Part model, mm, in its own coordinate system. A direction names the side the tool comes from. Round coordinates to 2 decimals unless told otherwise and drop trailing zeros. Write each loop counter-clockwise with the first axis right and the second up, starting at its lowest first coordinate (ties: lowest second). Pieces come first, ordered by that corner, then holes.
1) Drill centre lines: L1, parallel to Z at x = -0.5, y = -14.5; L2, parallel to Y at x = -0.7, z = 54.5; L3, parallel to Z at x = 1.3, y = -5.5. Where is each one in solid material? Low to high.
2) Saw through at B-B on z = 48. Write the cut outline in (x, y), and give its area (3 significant figures).
3) Flat gauge pins, fed straight in: pin 1 (1.6 mm diameter, centred on y = -5.02, z = 28.49, fed in from -X); pin 2 (1 mm diameter, centred on x = 1, y = 53, fed in from -Z); pin 3 (1 mm diameter, centred on x = -1, z = -19, fed in from +Y); pin 4 (1 mm diameter, centred on x = 2, z = -23.5, fed in from -Y). Where does each tip first touch, or does it go through?
4) Saw through at A-A on y = -34. Write the cut outline in (x, z).
5) Saw through at C-C on y = 45. Write the cut outline in (x, z), and give its area (3 significant figures).
6) Which spindle directions (+Z, -Z, +X, -X, +Y, -Y) get a long thin tool onto all of the face, cutting with end or side? Do faces 1 (the flat face through (0.042, -64.765, -1.144)), 2 (the cylindrical face through (0.042, 7.046, 60.318)), 3 (the flat face through (0.042, 23.317, -13.135)). Say none if no direction does.
```python
from build123d import *

# Parameters (mm, degrees)
SKETCH1_R                = 59
EXTRUDE1_DEPTH           = 3
EXTRUDE2_DEPTH           = 3
CIRPATTERN1_COUNT        = 6
F_2_0_2_DIAMETER_HOLE1_D = 2
F_2_0_2_DIAMETER_HOLE3_D = 2
F_2_0_2_DIAMETER_HOLE4_D = 2
CIRPATTERN2_COUNT        = 6
CIRPATTERN3_COUNT        = 5
CIRPATTERN3_ANGLE        = 240


with BuildPart() as part:
    # Sketch1 → Extrude1 (new, symmetric)
    with BuildSketch(Plane(origin=(0, 0, 0), x_dir=(0, 0, -1), z_dir=(1, 0, 0))):
        Circle(SKETCH1_R)
        Polygon((28.485808967, 5.022816688), (9.893017633, 27.180842557), (-18.592791334, 22.158025869), (-28.485808967, -5.022816688), (-9.893017633, -27.180842557), (18.592791334, -22.158025869), align=None, mode=Mode.SUBTRACT)
    extrude(amount=EXTRUDE1_DEPTH, both=True)

    # Sketch2 → Extrude2 (add, symmetric)
    with BuildSketch(Plane(origin=(0, 0, 0), x_dir=(0, 0, -1), z_dir=(1, 0, 0))):
        with BuildLine():
            Line((-2, 67.961805723), (-0.262709442, 61.478149092))
            ThreePointArc((-0.262709442, 61.478149092), (-0.58620663, 59.77173183), (-2.122608272, 58.961805723))
            ThreePointArc((-2.122608272, 58.961805723), (28.679663449, 51.560419941), (51.21368579, 29.294340542))
            ThreePointArc((51.21368579, 29.294340542), (36.791707484, 48.186627241), (17.927108603, 62.644803614))
            ThreePointArc((17.927108603, 62.644803614), (8.312130826, 66.609702921), (-2, 67.961805723))
        make_face()
    extrude2 = extrude(amount=EXTRUDE2_DEPTH, both=True)

    # CirPattern1: Extrude2 ×6 about axis
    cirpattern1_axis = Axis((0, 0, 0), (1, 0, 0))
    for i in range(1, CIRPATTERN1_COUNT):
        add(extrude2.rotate(cirpattern1_axis, i * 360 / CIRPATTERN1_COUNT))

    # Ø2.0 (2) Diameter Hole1 (through all)
    with Locations(Plane(origin=(3, 0, 0), x_dir=(0, 0, -1), z_dir=(1, 0, 0))):
        with Locations((9.893017633, 27.180842557), (28.485808967, 5.022816688), (18.592791334, -22.158025869), (-9.893017633, -27.180842557), (-28.485808967, -5.022816688), (-18.592791334, 22.158025869)):
            Hole(F_2_0_2_DIAMETER_HOLE1_D / 2)

    # Ø2.0 (2) Diameter Hole3 (through all)
    with Locations(Plane(origin=(3, 0, 0), x_dir=(0, 0, -1), z_dir=(1, 0, 0))):
        with Locations((16.304877281, 19.539485786)):
            f_2_0_2_diameter_hole3 = Hole(F_2_0_2_DIAMETER_HOLE3_D / 2)

    # Ø2.0 (2) Diameter Hole4 (through all)
    with Locations(Plane(origin=(3, 0, 0), x_dir=(0, 0, -1), z_dir=(1, 0, 0))):
        with Locations((22.395343124, 12.281151237)):
            f_2_0_2_diameter_hole4 = Hole(F_2_0_2_DIAMETER_HOLE4_D / 2)

    # CirPattern2: Ø2.0 (2) Diameter Hole3 ×6 about axis
    cirpattern2_axis = Axis((0, 0, 0), (1, 0, 0))
    for i in range(1, CIRPATTERN2_COUNT):
        add(f_2_0_2_diameter_hole3.rotate(cirpattern2_axis, i * 360 / CIRPATTERN2_COUNT), mode=Mode.SUBTRACT)

    # CirPattern3: Ø2.0 (2) Diameter Hole4 ×5 about axis
    cirpattern3_axis = Axis((0, 0, 0), (-1, 0, 0))
    for i in range(1, CIRPATTERN3_COUNT):
        add(f_2_0_2_diameter_hole4.rotate(cirpattern3_axis, i * CIRPATTERN3_ANGLE / (CIRPATTERN3_COUNT - 1)), mode=Mode.SUBTRACT)


solid = part.part
```
Completed:
1. L1: z = -58.03 to -21.38, 20.53 to 63.21
1. L2: y = -32.36 to 23.03, 30.81 to 39.5
1. L3: z = -60.71 to -24.66, 29.36 to 62.65
2. outline: (-3, -34.49) - (3, -34.49) - (3, 45.13) - (-3, 45.13) - close
2. area: 478 mm2
3. pin 1: passes through
3. pin 2: stops at z = -32.17
3. pin 3: stops at y = 62.31
3. pin 4: stops at y = -56.04
4. outline: (-3, -58.78) - (3, -58.78) - (3, 48.33) - (-3, 48.33) - close; (-3, 56.14) - (3, 56.14) - (3, 58.79) - (-3, 58.79) - close
5. outline: (-3, -39.82) - (3, -39.82) - (3, 48.18) - (-3, 48.18) - close
5. area: 528 mm2
6. face 1: -Z, +X, -X
6. face 2: +Z, +X, -X
6. face 3: +X, -X
